The listing builds one solid part. Answer for the finished solid, in the listing's coordinates (mm). Face numbers are marked on the shaded views. Give positions to 0.01 mm unless a question says otherwise; leave off trailing zeros. Write each loop counter-clockwise with the first axis right and the second up, starting at its lowest first coordinate (ties: lowest second). Pieces come first, ordered by that corner, then holes. Notation, with made-up numbers: (-25, 77.5) - (5, 77.5) arc R24 ccw to (5, 108.5) - close; hole circle Ø7 at (57.25, 44). An arc over 180 degrees is marked (long way). Return JSON: item names as keys, results as strings.
from build123d import *


with BuildPart() as part:
    # Sketch1 → Revolve1 (revolve)
    with BuildSketch(Plane.XY, mode=Mode.PRIVATE) as revolve1_sk:
        with BuildLine():
            Line((8.94427191, 37), (13.5, 37))
            ThreePointArc((13.5, 37), (14.914213562, 36.414213562), (15.5, 35))
            Line((15.5, 35), (15.5, 25))
            Line((15.5, 25), (-15.5, 25))
            Line((-15.5, 25), (-15.5, 35))
            ThreePointArc((-15.5, 35), (-14.914213562, 36.414213562), (-13.5, 37))
            Line((-13.5, 37), (-8.94427191, 37))
            ThreePointArc((-8.94427191, 37), (0, 33), (8.94427191, 37))
        make_face()
    revolve(revolve1_sk.sketch.rotate(Axis((0, 0, 0), (1, 0, 0)), 90), axis=Axis((0, 0, 0), (1, 0, 0)))


solid = part.part
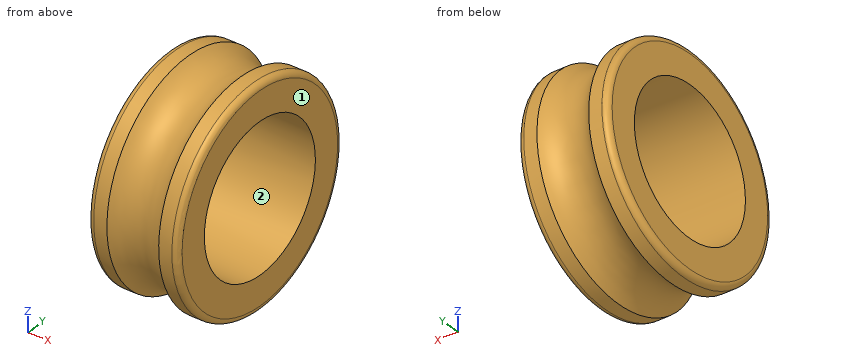
Item 1: A cutting plane is placed at C-C on x = 10.5. Determine the outline of the cut face in (y, z).
Answer below:
{"outline": "circle Ø74 at (0, 0); hole circle Ø50 at (0, 0)"}
Item 2: The mould has two halves that part along Z. Classify the marked faces 1 and 2: +Z half, -Z half, draft (parallel to the pull), parting line (faces both ways), or undercut.
Answer below:
{"face 1": "draft", "face 2": "undercut"}
Item 3: Flat-ended cylindrical pins translate along their axes: P1, Ø2, axis at x = 11, y = -9, coming from the -Z side; P2, Ø5, axis at x = -6, z = 6, coming from the +Y side; P3, Ø12, axis at x = 11, z = 0, coming from the +Y side. Find the tip coordinate at first contact, or state that the pin passes through.
Answer below:
{"P1": "stops at z = -36.12", "P2": "stops at y = 36.07", "P3": "stops at y = 37"}
Item 4: Consider L1, parallel to Y at x = 9, z = 0; L2, parallel to Y at x = 2.5, z = 0; L3, parallel to Z at x = -4, y = 3. Determine where each line is inside the solid, lowest interval first.
Answer below:
{"L1": "y = -37 to -25, 25 to 37", "L2": "y = -33.26 to -25, 25 to 33.26", "L3": "z = -33.55 to -24.82, 24.82 to 33.55"}
Item 5: A cutting plane is placed at A-A on z = 0. Determine the outline of the cut face in (x, y), then the cut area to 3 significant figures.
Answer below:
{"outline": "(-15.5, -35) arc R2 ccw to (-13.5, -37) - (-8.94, -37) arc R12 cw to (8.94, -37) - (13.5, -37) arc R2 ccw to (15.5, -35) - (15.5, -25) - (-15.5, -25) - close; (-15.5, 25) - (15.5, 25) - (15.5, 35) arc R2 ccw to (13.5, 37) - (8.94, 37) arc R12 cw to (-8.94, 37) - (-13.5, 37) arc R2 ccw to (-15.5, 35) - close", "area": "641 mm²"}
Item 6: A cutting plane is placed at D-D on x = 6. Determine the outline of the cut face in (y, z).
Answer below:
{"outline": "circle Ø69.22 at (0, 0); hole circle Ø50 at (0, 0)"}
